```python
from build123d import *

# Parameters (mm, degrees)
CROQUIS1_R              = 16.75
SALIENTE_EXTRUIR1_DEPTH = 10
CROQUIS2_R              = 1.5
CORTAR_EXTRUIR1_DEPTH   = 67


with BuildPart() as part:
    # Croquis1 → Saliente-Extruir1 (new body)
    with BuildSketch(Plane.XY):
        with BuildLine():
            Line((-23.5, -5), (-19.364916731, -5))
            ThreePointArc((-19.364916731, -5), (0, -20), (19.364916731, -5))
            Line((19.364916731, -5), (23.5, -5))
            Line((23.5, -5), (23.5, 5))
            Line((23.5, 5), (19.364916731, 5))
            ThreePointArc((19.364916731, 5), (0, 20), (-19.364916731, 5))
            Line((-19.364916731, 5), (-23.5, 5))
            Line((-23.5, 5), (-23.5, -5))
        make_face()
        Circle(CROQUIS1_R, mode=Mode.SUBTRACT)
    extrude(amount=SALIENTE_EXTRUIR1_DEPTH)

    # Croquis2 → Cortar-Extruir1 (cut)
    with BuildSketch(Plane(origin=(23.5, 0, 0), x_dir=(0, 0, -1), z_dir=(1, 0, 0))):
        with Locations(Location((-5, 0, 0), (0, 0, 90))):
            Circle(CROQUIS2_R)
    extrude(amount=-CORTAR_EXTRUIR1_DEPTH, mode=Mode.SUBTRACT)


solid = part.part
```
Geometry: final body of the model. Coordinates: model frame, mm. A direction names the side the tool comes from. Round coordinates to 2 decimals unless told otherwise and drop trailing zeros. Loops run counter-clockwise (first coordinate to the right, second up) from the corner with the lowest first, then second, coordinate; pieces in that order, holes last. Notation, with made-up numbers: (25.25, -9.75) -> (77.25, -9.75) arc R5 cw to (77.25, -2.75) -> close; hole circle Ø9 at (-29.75, -39.5). An arc over 180 degrees is marked (long way). Use one line per item in the form item = value.
Item 1: Cut plane C-C on y = 0. Output: boundary loops of the cut face in (x, z), then the cut area to 3 significant figures.
Evaluation:
outline = (-23.5, 0) -> (-16.75, 0) -> (-16.75, 3.5) -> (-23.5, 3.5) -> close; (-23.5, 6.5) -> (-16.75, 6.5) -> (-16.75, 10) -> (-23.5, 10) -> close; (16.75, 0) -> (23.5, 0) -> (23.5, 3.5) -> (16.75, 3.5) -> close; (16.75, 6.5) -> (23.5, 6.5) -> (23.5, 10) -> (16.75, 10) -> close
area = 94.5 mm2
Item 2: Cut plane A-A on x = 0. Output: boundary loops of the cut face in (y, z), then the cut area to 3 significant figures.
Evaluation:
outline = (-20, 0) -> (-16.75, 0) -> (-16.75, 10) -> (-20, 10) -> close; (16.75, 0) -> (20, 0) -> (20, 10) -> (16.75, 10) -> close
area = 65.0 mm2
Item 3: Material intervals for probe 1 along Z at (x, y) = (-20.75, 0); probe 2 along X at (y, z) = (0, 2.75); probe 3 along Y at (x, z) = (-20.25, 5), sorted ascending.
Evaluation:
probe_1 = 0 to 3.5, 6.5 to 10
probe_2 = -23.5 to -16.75, 16.75 to 23.5
probe_3 = -5 to -1.5, 1.5 to 5
Item 4: Cut plane D-D on z = 1.75. Output: boundary loops of the cut face in (x, y).
Evaluation:
outline = (-23.5, -5) -> (-19.36, -5) arc R20 ccw to (19.36, -5) -> (23.5, -5) -> (23.5, 5) -> (19.36, 5) arc R20 ccw to (-19.36, 5) -> (-23.5, 5) -> close; hole circle Ø33.5 at (0, 0)
Item 5: Cut plane B-B on z = 5. Output: boundary loops of the cut face in (x, y), then the cut area to 3 significant figures.
Evaluation:
outline = (-23.5, -5) -> (-19.36, -5) arc R20 ccw to (19.36, -5) -> (23.5, -5) -> (23.5, -1.5) -> (16.68, -1.5) arc R16.75 cw to (-16.68, -1.5) -> (-23.5, -1.5) -> close; (-23.5, 1.5) -> (-16.68, 1.5) arc R16.75 cw to (16.68, 1.5) -> (23.5, 1.5) -> (23.5, 5) -> (19.36, 5) arc R20 ccw to (-19.36, 5) -> (-23.5, 5) -> close
area = 409 mm2
Item 6: Draft query along Y for faces 4 (the flat face through (-5.3, -16.2, 10)), 5 (the flat face through (21, 5, 5)), 6 (the cylindrical face through (15.47, -6.42, 4.93)), 7 (the flat face through (-21, -5, 5)). Return one class per face: released by +Y, released by -Y, zero draft, split by the parting line, or undercut.
Evaluation:
face_4 = zero draft
face_5 = released by +Y
face_6 = undercut
face_7 = released by -Y
Item 7: Contact query for flat-ended pins moving along their axis: pin 1 Ø4 at (x, z) = (15.5, 3) entering from +Y; pin 2 Ø3.5 at (x, z) = (21.5, 4.5) entering from -Y; pin 3 Ø1 at (x, z) = (4, 6) entering from +Y. Output: stop coordinate, or through.
Evaluation:
pin_1 = 14.76
pin_2 = -5
pin_3 = 19.69
Item 8: Access query for faces 1 (the flat face through (23.5, -1.2, 3.8)), 2 (the flat face through (21, -5, 5)), 3 (the flat face through (-21, 5, 5)). Directions: +Z, -Z, +X, -X, +Y, -Y. A direction counts if a zero-diameter tool reaches every point of the face in a straight line with its end or side. Return the directions, or none.
Evaluation:
face_1 = +Z, -Z, +X, +Y, -Y
face_2 = +Z, -Z, +X, -Y
face_3 = +Z, -Z, -X, +Y
